```python
from build123d import *

# Parameters (mm, degrees)
SKETCH1_R               = 20
SKETCH1_R_2             = 4
SKETCH1_R_3             = 1.5
BOSS_EXTRUDE1_DEPTH     = 5
SKETCH2_R               = 7
SKETCH2_R_2             = 4
BOSS_EXTRUDE2_DEPTH     = 10
SKETCH3_R               = 50
SKETCH3_R_2             = 4
BOSS_EXTRUDE3_DEPTH     = 2
CUT_EXTRUDE1_START      = -2
CUT_EXTRUDE1_DEPTH      = 2
CUT_EXTRUDE2_DEPTH      = 72.944422994
CUT_EXTRUDE2_DEPTH_BACK = 72.944422994
SKETCH5_R               = 1.5


with BuildPart() as part:
    # Sketch1 → Boss-Extrude1 (new body)
    with BuildSketch(Plane.XY):
        Circle(SKETCH1_R)
        Circle(SKETCH1_R_2, mode=Mode.SUBTRACT)
        with Locations((-10.061951403, 10.061951403)):
            Circle(SKETCH1_R_3, mode=Mode.SUBTRACT)
        with Locations(Location((10.061951403, 10.061951403, 0), (0, 0, 180))):
            Circle(SKETCH1_R_3, mode=Mode.SUBTRACT)
        with Locations((10.061951403, -10.061951403)):
            Circle(SKETCH1_R_3, mode=Mode.SUBTRACT)
        with Locations(Location((-10.061951403, -10.061951403, 0), (0, 0, 180))):
            Circle(SKETCH1_R_3, mode=Mode.SUBTRACT)
    extrude(amount=BOSS_EXTRUDE1_DEPTH)

    # Sketch2 → Boss-Extrude2 (add)
    with BuildSketch(Plane.XY.offset(5)):
        Circle(SKETCH2_R)
        Circle(SKETCH2_R_2, mode=Mode.SUBTRACT)
    extrude(amount=BOSS_EXTRUDE2_DEPTH)

    # Sketch3 → Boss-Extrude3 (add)
    with BuildSketch(Plane.XY.offset(5)):
        Circle(SKETCH3_R)
        Circle(SKETCH3_R_2, mode=Mode.SUBTRACT)
    extrude(amount=BOSS_EXTRUDE3_DEPTH)

    # Sketch4 → Cut-Extrude1 (cut)
    with BuildSketch(Plane.XY.offset(7).offset(CUT_EXTRUDE1_START)):
        with BuildLine():
            Line((-7, 49.507575178), (-7, 34.507575178))
            ThreePointArc((-7, 34.507575178), (0, 27.507575178), (7, 34.507575178))
            Line((7, 34.507575178), (7, 49.507575178))
            ThreePointArc((7, 49.507575178), (0, 50), (-7, 49.507575178))
        make_face()
        with BuildLine():
            Line((39.374817784, 30.815965415), (26.384436727, 23.315965415))
            ThreePointArc((26.384436727, 23.315965415), (23.822258901, 13.753787589), (33.384436727, 11.191609762))
            Line((33.384436727, 11.191609762), (46.374817784, 18.691609762))
            ThreePointArc((46.374817784, 18.691609762), (43.301270189, 25), (39.374817784, 30.815965415))
        make_face()
        with BuildLine():
            Line((46.374817784, -18.691609762), (33.384436727, -11.191609762))
            ThreePointArc((33.384436727, -11.191609762), (23.822258901, -13.753787589), (26.384436727, -23.315965415))
            Line((26.384436727, -23.315965415), (39.374817784, -30.815965415))
            ThreePointArc((39.374817784, -30.815965415), (43.301270189, -25), (46.374817784, -18.691609762))
        make_face()
        with BuildLine():
            Line((7, -49.507575178), (7, -34.507575178))
            ThreePointArc((7, -34.507575178), (0, -27.507575178), (-7, -34.507575178))
            Line((-7, -34.507575178), (-7, -49.507575178))
            ThreePointArc((-7, -49.507575178), (0, -50), (7, -49.507575178))
        make_face()
        with BuildLine():
            Line((-39.374817784, -30.815965415), (-26.384436727, -23.315965415))
            ThreePointArc((-26.384436727, -23.315965415), (-23.822258901, -13.753787589), (-33.384436727, -11.191609762))
            Line((-33.384436727, -11.191609762), (-46.374817784, -18.691609762))
            ThreePointArc((-46.374817784, -18.691609762), (-43.301270189, -25), (-39.374817784, -30.815965415))
        make_face()
        with BuildLine():
            Line((-46.374817784, 18.691609762), (-33.384436727, 11.191609762))
            ThreePointArc((-33.384436727, 11.191609762), (-23.822258901, 13.753787589), (-26.384436727, 23.315965415))
            Line((-26.384436727, 23.315965415), (-39.374817784, 30.815965415))
            ThreePointArc((-39.374817784, 30.815965415), (-43.301270189, 25), (-46.374817784, 18.691609762))
        make_face()
    extrude(amount=CUT_EXTRUDE1_DEPTH, mode=Mode.SUBTRACT)

    # Sketch5 → Cut-Extrude2 (cut, two sides: drawn at the far end of the back side and taken through both)
    with BuildSketch(Plane(origin=(0, 0, 0), x_dir=(-1, 0, 0), z_dir=(0, 0, -1)).offset(-CUT_EXTRUDE2_DEPTH_BACK)):
        with Locations((-10.061951403, 10.061951403)):
            Circle(SKETCH5_R)
        with Locations(Location((-10.061951403, -10.061951403, 0), (0, 0, 180))):
            Circle(SKETCH5_R)
        with Locations(Location((10.061951403, 10.061951403, 0), (0, 0, 180))):
            Circle(SKETCH5_R)
        with Locations((10.061951403, -10.061951403)):
            Circle(SKETCH5_R)
    extrude(amount=CUT_EXTRUDE2_DEPTH + CUT_EXTRUDE2_DEPTH_BACK, mode=Mode.SUBTRACT)


solid = part.part
```
Model file for the job. Use its own axes, mm. A direction names the side the tool comes from. Coordinates: 2 decimals unless noted, no trailing zeros. Write each loop counter-clockwise with the first axis right and the second up, starting at its lowest first coordinate (ties: lowest second). Pieces come first, ordered by that corner, then holes. Notation, with made-up numbers: (-0.75, 2.25) - (10.25, 2.25) arc R19 cw to (10.25, 17.25) - close; hole circle Ø6 at (-32, -21). An arc over 180 degrees is marked (long way). Use a Markdown table: item, result. Add a question column.
Item 1: Band-saw the part on A-A, the plane y = 0. Write the cut outline in (x, z).
Item 2: Two-plate mould, pull along X, no slides. Class faces 1 (the face through (-1, -10, 7)), 2 (the face through (24.767, -43.435, 5.986)), 3 (the face through (9, 9, 4)): pulls with the +X half, pulls with the -X half, needs draft (parallel to the pull), parting line crosses it, or undercut.
Item 3: Band-saw the part on B-B, the plane x = 0. Write the cut outline in (y, z), and give its area (3 significant figures).
Item 4: Drop flat-ended pins along their axis: pin 1 (4 mm diameter, centred on x = -22.5, y = -2.5, fed in from -Z); pin 2 (10 mm diameter, centred on x = -23.5, y = 17, fed in from +Z); pin 3 (1 mm diameter, centred on y = 41, z = 5.5, fed in from -X). Give the stop position or say it passes through.
Item 5: Drill centre lines: line 1 along Y through (x, z) = (0, 7.5); line 2 along Z through (x, y) = (18.5, -40); line 3 along Z through (x, y) = (-17, 2.5). Where is each one in solid material? Low to high.
Item 6: 3-axis set-ups, long thin cutter, end or side, ignore diameter. For faces 4 (the face through (32.97, 27.12, 5.99)), 5 (the face through (-39.971, 14.994, 5.986)), 6 (the face through (-32.97, -27.12, 5.99)), 7 (the face through (6.466, -2.681, 10.944)), 8 (the face through (-4.336, -19.524, 2.465)): which of +Z, -Z, +X, -X, +Y, -Y reach the whole face in a straight line?
Item 7: Band-saw the part on D-D, the plane z = 1.25. Write the cut outline in (x, y), and give its area (3 significant figures).
Item 8: Band-saw the part on C-C, the plane x = 29.5. Write the cut outline in (y, z).
A:
| question | item | result |
|---|---|---|
| 1 | outline | (-50, 5) - (-20, 5) - (-20, 0) - (-4, 0) - (-4, 15) - (-7, 15) - (-7, 7) - (-50, 7) - close; (4, 0) - (20, 0) - (20, 5) - (50, 5) - (50, 7) - (7, 7) - (7, 15) - (4, 15) - close |
| 2 | face 1 | needs draft |
| 2 | face 2 | pulls with the +X half |
| 2 | face 3 | undercut |
| 3 | outline | (-27.51, 5) - (-20, 5) - (-20, 0) - (-4, 0) - (-4, 15) - (-7, 15) - (-7, 7) - (-27.51, 7) - close; (4, 0) - (20, 0) - (20, 5) - (27.51, 5) - (27.51, 7) - (7, 7) - (7, 15) - (4, 15) - close |
| 3 | area | 302 mm² |
| 4 | pin 1 | stops at z = 5 |
| 4 | pin 2 | stops at z = 7 |
| 4 | pin 3 | stops at x = -29.32 |
| 5 | line 1 | y = -7 to -4, 4 to 7 |
| 5 | line 2 | z = 5 to 7 |
| 5 | line 3 | z = 0 to 7 |
| 6 | face 4 | +Z, -Z, +X |
| 6 | face 5 | +Z, -Z |
| 6 | face 6 | +Z, -Z, -X |
| 6 | face 7 | +Z |
| 6 | face 8 | -Z |
| 7 | outline | circle Ø40 at (0, 0); hole circle Ø3 at (-10.06, -10.06); hole circle Ø3 at (-10.06, 10.06); hole circle Ø8 at (0, 0); hole circle Ø3 at (10.06, -10.06); hole circle Ø3 at (10.06, 10.06) |
| 7 | area | 1,180 mm² |
| 8 | outline | (-40.37, 5) - (-25.11, 5) - (-25.11, 7) - (-40.37, 7) - close; (-10.26, 5) - (10.26, 5) - (10.26, 7) - (-10.26, 7) - close; (25.11, 5) - (40.37, 5) - (40.37, 7) - (25.11, 7) - close |
